```python
from build123d import *

# Parameters (mm, degrees)
SKETCH1_R           = 44
SKETCH1_R_2         = 42.65
BOSS_EXTRUDE1_DEPTH = 11.5
BOSS_EXTRUDE2_START = 2
SKETCH1_2_R         = 44
SKETCH1_2_R_2       = 34
BOSS_EXTRUDE2_DEPTH = 2
BOSS_EXTRUDE3_DEPTH = 6
SKETCH7_R           = 42.65
SKETCH7_R_2         = 39.5
BOSS_EXTRUDE4_DEPTH = 1
SKETCH8_R           = 5.25
SKETCH8_R_2         = 0.85
SKETCH8_R_3         = 2.6
CUT_EXTRUDE3_DEPTH  = 10
SKETCH9_R           = 12.5
CUT_EXTRUDE4_DEPTH  = 3
CHAMFER1_SIZE       = 1.8
CHAMFER1_SIZE2      = 3.117691454
BOSS_EXTRUDE5_START = -2
SKETCH11_R          = 5
SKETCH11_R_2        = 2.6
BOSS_EXTRUDE5_DEPTH = 2


with BuildPart() as part:
    # Sketch1 → Boss-Extrude1 (new body)
    with BuildSketch(Plane(origin=(0, 0, 0), x_dir=(0, 0, -1), z_dir=(1, 0, 0))):
        Circle(SKETCH1_R)
        Circle(SKETCH1_R_2, mode=Mode.SUBTRACT)
    extrude(amount=-BOSS_EXTRUDE1_DEPTH)

    # Sketch1_2 → Boss-Extrude2 (add)
    with BuildSketch(Plane(origin=(0, 0, 0), x_dir=(0, 0, -1), z_dir=(1, 0, 0)).offset(BOSS_EXTRUDE2_START)):
        Circle(SKETCH1_2_R)
        Circle(SKETCH1_2_R_2, mode=Mode.SUBTRACT)
    extrude(amount=-BOSS_EXTRUDE2_DEPTH)

    # Sketch5 → Boss-Extrude3 (add)
    with BuildSketch(Plane(origin=(-2, 0, 0), x_dir=(0, 0, -1), z_dir=(1, 0, 0))):
        with BuildLine():
            Line((-25, -36.20773398), (-25, -86))
            Line((-25, -86), (25, -86))
            Line((25, -86), (25, -36.20773398))
            ThreePointArc((25, -36.20773398), (0, -44), (-25, -36.20773398))
        make_face()
    extrude(amount=-BOSS_EXTRUDE3_DEPTH)

    # Sketch7 → Boss-Extrude4 (add)
    with BuildSketch(Plane.ZY):
        with Locations(Location((0, 0, 0), (0, 0, 180))):
            Circle(SKETCH7_R)
        Circle(SKETCH7_R_2, mode=Mode.SUBTRACT)
    extrude(amount=BOSS_EXTRUDE4_DEPTH)

    # Sketch8 → Cut-Extrude3 (cut)
    with BuildSketch(Plane(origin=(-2, 0, 0), x_dir=(0, 0, -1), z_dir=(1, 0, 0))):
        with Locations((0, -57.5)):
            Circle(SKETCH8_R)
        with Locations((0, -64.86)):
            Circle(SKETCH8_R_2)
        with Locations((-10, -76)):
            Circle(SKETCH8_R_3)
        with Locations((10, -76)):
            Circle(SKETCH8_R_3)
    extrude(amount=-CUT_EXTRUDE3_DEPTH, mode=Mode.SUBTRACT)

    # Sketch9 → Cut-Extrude4 (cut)
    with BuildSketch(Plane.ZY.offset(8)):
        with Locations((0, -57.5)):
            Circle(SKETCH9_R)
    extrude(amount=-CUT_EXTRUDE4_DEPTH, mode=Mode.SUBTRACT)

    # Chamfer1
    chamfer1_edges = [part.edges().sort_by_distance(p)[0] for p in [
        (2, 0, 34),
    ]]
    chamfer1_side = [part.faces().sort_by_distance(p)[0] for p in [
        (1, 0, 34),
    ]]
    chamfer(chamfer1_edges, length=CHAMFER1_SIZE, length2=CHAMFER1_SIZE2, reference=chamfer1_side[0])

    # Sketch11 → Boss-Extrude5 (add)
    # profile 1 of 2: a face of its own
    with BuildSketch(Plane.ZY.offset(2).offset(BOSS_EXTRUDE5_START)):
        with Locations((-10, -76)):
            Circle(SKETCH11_R)
        with Locations(Location((-10, -76, 0), (0, 0, 180))):
            Circle(SKETCH11_R_2, mode=Mode.SUBTRACT)
    # profile 2 of 2: a face of its own
    with BuildSketch(Plane.ZY.offset(2).offset(BOSS_EXTRUDE5_START)):
        with Locations((10, -76)):
            Circle(SKETCH11_R)
        with Locations(Location((10, -76, 0), (0, 0, 180))):
            Circle(SKETCH11_R_2, mode=Mode.SUBTRACT)
    extrude(amount=BOSS_EXTRUDE5_DEPTH)


solid = part.part
```
Work out the finished part from the listing and answer in its coordinate system (mm). A direction names the side the tool comes from. Round coordinates to 2 decimals unless told otherwise and drop trailing zeros. Loops run counter-clockwise (first coordinate to the right, second up) from the corner with the lowest first, then second, coordinate; pieces in that order, holes last. Notation, with made-up numbers: M -11,60 L 47,60 A9 cw 47,77 Z; hole C 38,86.25 d10. An arc over 180 degrees is marked long. Use CSV: the item, a comma, the result in double quotes.
Q1. Section B-B, the plane y = -76 is taken. Determine the outline of the cut face in (x, z), then the cut area to 3 significant figures.
Determined:
outline,"M -8,-25 L -2,-25 L -2,-15 L 0,-15 L 0,-12.6 L -8,-12.6 Z; M -8,-7.4 L 0,-7.4 L 0,-5 L -2,-5 L -2,5 L 0,5 L 0,7.4 L -8,7.4 Z; M -8,12.6 L 0,12.6 L 0,15 L -2,15 L -2,25 L -8,25 Z"
area,"257 mm2"
Q2. Section C-C, the plane y = -57.5 is taken. Determine the outline of the cut face in (x, z).
Determined:
outline,"M -8,-25 L -2,-25 L -2,-5.25 L -5,-5.25 L -5,-12.5 L -8,-12.5 Z; M -8,12.5 L -5,12.5 L -5,5.25 L -2,5.25 L -2,25 L -8,25 Z"
Q3. Consider L1, parallel to Y at x = -3.2, z = 0; L2, parallel to Z at x = -2.7, y = -64.86; L3, parallel to Y at x = 0.15, z = 0. Determine where each line is inside the solid, lowest interval first.
Determined:
L1,"-86 to -65.71, -64.01 to -62.75, -52.25 to -42.65, 42.65 to 44"
L2,"-25 to -0.85, 0.85 to 25"
L3,"-44 to -34, 34 to 44"
Q4. A tool of negligible diameter and unlimited length cuts with its end or side. For faces 4 (the cylindrical face through (-0.49, 26.7, -29.11)), 5 (the flat face through (0, -78, -8)), 6 (the cylindrical face through (-0.99, -80.88, 8.92)), from which of +Z, -Z, +X, -X, +Y, -Y can it reach the whole face along a straight path? Write none if from no direction.
Determined:
face 4,"-X"
face 5,"+Z, -Z, +X, -Y"
face 6,"+X"
Q5. Section D-D, the plane z = 3 is taken. State how many separate pieces and enclosed holes the cut face has, then the cut area to 3 significant figures.
Determined:
separate pieces,"3"
enclosed holes,"0"
area,"226 mm2"
Q6. Each of these flat-tipped pins is pushed along its axis until it touches: pin 1 (6 mm diameter, centred on x = -7, y = -45, fed in from -Z); pin 2 (11 mm diameter, centred on y = -78, z = -8, fed in from +X); pin 3 (7.5 mm diameter, centred on y = -61, z = -6, fed in from -X). Where does it stop, or does it pass through?
Determined:
pin 1,"z = -25"
pin 2,"x = 0"
pin 3,"x = -5"
Q7. The mould has two halves that part along Y. Classify faces 1 (the flat face through (-5, -86, 0)), 2 (the flat face through (-5, -61, -25)), 3 (the flat face through (0, 29.4, -17.4)): pulls with the +Y half, pulls with the -Y half, needs draft (parallel to the pull), parting line crosses it, or undercut.
Determined:
face 1,"pulls with the -Y half"
face 2,"needs draft"
face 3,"undercut"
Q8. Section A-A, the plane y = 0 is taken. Determine the outline of the cut face in (x, z).
Determined:
outline,"M -11.5,-44 L 2,-44 L 2,-37.12 L 0.2,-34 L 0,-34 L 0,-39.5 L -1,-39.5 L -1,-42.65 L -11.5,-42.65 Z; M -11.5,42.65 L -1,42.65 L -1,39.5 L 0,39.5 L 0,34 L 0.2,34 L 2,37.12 L 2,44 L -11.5,44 Z"
